```python
from build123d import *

# Parameters (mm, degrees)
F0_W     = 40
F0_H     = 20
F0_R     = 7.096656
F1_DEPTH = 25
F2_R     = 5
F3_DEPTH = 25


with BuildPart() as f1:
    # F0 (on Top) → F1 (new body)
    with BuildSketch(Plane.XY):
        with BuildLine():
            ThreePointArc((-133.453285, 45.853535), (-140.524353, 42.924603), (-143.453285, 35.853535))
            Line((-143.453285, 35.853535), (-143.453285, -36.596949))
            ThreePointArc((-143.453285, -36.596949), (-140.524353, -43.668016), (-133.453285, -46.596949))
            Line((-133.453285, -46.596949), (-93.023613, -46.596949))
            Line((-93.023613, -46.596949), (-93.023613, -53.490194))
            ThreePointArc((-93.023613, -53.490194), (-90.680467, -59.147049), (-85.023613, -61.490194))
            Line((-85.023613, -61.490194), (12.305611, -61.490194))
            Line((12.305611, -61.490194), (12.305611, -52.104292))
            Line((12.305611, -52.104292), (35.921164, -52.104292))
            ThreePointArc((35.921164, -52.104292), (39.456698, -50.639826), (40.921164, -47.104292))
            Line((40.921164, -47.104292), (40.921164, 45.453855))
            ThreePointArc((40.921164, 45.453855), (39.456698, 48.989389), (35.921164, 50.453855))
            Line((35.921164, 50.453855), (12.305611, 50.453855))
            Line((12.305611, 50.453855), (12.305611, 69.478564))
            Line((12.305611, 69.478564), (-88.023613, 69.478564))
            ThreePointArc((-88.023613, 69.478564), (-91.559147, 68.014098), (-93.023613, 64.478564))
            Line((-93.023613, 64.478564), (-93.023613, 45.853535))
            Line((-93.023613, 45.853535), (-133.453285, 45.853535))
        make_face()
        with BuildLine():
            Line((-138.153107, -41.573759), (-138.153107, -21.573759))
            Line((-138.153107, -21.573759), (-98.153107, -21.573759))
            Line((-98.153107, -21.573759), (-98.153107, -38.573759))
            ThreePointArc((-98.153107, -38.573759), (-99.031787, -40.695079), (-101.153107, -41.573759))
            Line((-101.153107, -41.573759), (-138.153107, -41.573759))
        make_face(mode=Mode.SUBTRACT)
        with Locations((-118.975651, -3.308505)):
            Rectangle(F0_W, F0_H, mode=Mode.SUBTRACT)
        with Locations((26.162848, -33.166352)):
            Circle(F0_R, mode=Mode.SUBTRACT)
        with BuildLine():
            Line((-76.998904, -36.091934), (-76.998904, 0))
            Line((-76.998904, 0), (0, 0))
            Line((0, 0), (0, -36.091934))
            ThreePointArc((0, -36.091934), (-1.464466, -39.627468), (-5, -41.091934))
            Line((-5, -41.091934), (-71.998904, -41.091934))
            ThreePointArc((-71.998904, -41.091934), (-75.534438, -39.627468), (-76.998904, -36.091934))
        make_face(mode=Mode.SUBTRACT)
        with Locations((25.7, 0.3)):
            Circle(F0_R, mode=Mode.SUBTRACT)
        with BuildLine():
            Line((-138.975651, 11.789608), (-138.975651, 31.789608))
            Line((-138.975651, 31.789608), (-103.975651, 31.789608))
            ThreePointArc((-103.975651, 31.789608), (-100.440117, 30.325142), (-98.975651, 26.789608))
            Line((-98.975651, 26.789608), (-98.975651, 11.789608))
            Line((-98.975651, 11.789608), (-138.975651, 11.789608))
        make_face(mode=Mode.SUBTRACT)
        with BuildLine():
            ThreePointArc((-77.227831, 41.128273), (-75.763365, 44.663807), (-72.227831, 46.128273))
            Line((-72.227831, 46.128273), (-5, 46.128273))
            ThreePointArc((-5, 46.128273), (-1.464466, 44.663807), (0, 41.128273))
            Line((0, 41.128273), (0, 17.970568))
            Line((0, 17.970568), (-77.227831, 17.970568))
            Line((-77.227831, 17.970568), (-77.227831, 41.128273))
        make_face(mode=Mode.SUBTRACT)
        with Locations((25.237152, 33.766352)):
            Circle(F0_R, mode=Mode.SUBTRACT)
    extrude(amount=F1_DEPTH)

    # F2
    f2_edges = [f1.edges().sort_by_distance(p)[0] for p in [
        (12.305611, -61.490194, 12.5),
        (-85.023613, -61.490194, 12.5),
    ]]
    fillet(f2_edges, radius=F2_R)

    # F0 (on Top) → F3 (join)
    with BuildSketch(Plane.XY):
        with BuildLine():
            ThreePointArc((-133.453285, 45.853535), (-140.524353, 42.924603), (-143.453285, 35.853535))
            Line((-143.453285, 35.853535), (-143.453285, -36.596949))
            ThreePointArc((-143.453285, -36.596949), (-140.524353, -43.668016), (-133.453285, -46.596949))
            Line((-133.453285, -46.596949), (-93.023613, -46.596949))
            Line((-93.023613, -46.596949), (-93.023613, -53.490194))
            ThreePointArc((-93.023613, -53.490194), (-90.680467, -59.147049), (-85.023613, -61.490194))
            Line((-85.023613, -61.490194), (12.305611, -61.490194))
            Line((12.305611, -61.490194), (12.305611, -52.104292))
            Line((12.305611, -52.104292), (35.921164, -52.104292))
            ThreePointArc((35.921164, -52.104292), (39.456698, -50.639826), (40.921164, -47.104292))
            Line((40.921164, -47.104292), (40.921164, 45.453855))
            ThreePointArc((40.921164, 45.453855), (39.456698, 48.989389), (35.921164, 50.453855))
            Line((35.921164, 50.453855), (12.305611, 50.453855))
            Line((12.305611, 50.453855), (12.305611, 69.478564))
            Line((12.305611, 69.478564), (-88.023613, 69.478564))
            ThreePointArc((-88.023613, 69.478564), (-91.559147, 68.014098), (-93.023613, 64.478564))
            Line((-93.023613, 64.478564), (-93.023613, 45.853535))
            Line((-93.023613, 45.853535), (-133.453285, 45.853535))
        make_face()
        with BuildLine():
            Line((-138.153107, -41.573759), (-138.153107, -21.573759))
            Line((-138.153107, -21.573759), (-98.153107, -21.573759))
            Line((-98.153107, -21.573759), (-98.153107, -38.573759))
            ThreePointArc((-98.153107, -38.573759), (-99.031787, -40.695079), (-101.153107, -41.573759))
            Line((-101.153107, -41.573759), (-138.153107, -41.573759))
        make_face(mode=Mode.SUBTRACT)
        with Locations((-118.975651, -3.308505)):
            Rectangle(F0_W, F0_H, mode=Mode.SUBTRACT)
        with Locations((26.162848, -33.166352)):
            Circle(F0_R, mode=Mode.SUBTRACT)
        with BuildLine():
            Line((-76.998904, -36.091934), (-76.998904, 0))
            Line((-76.998904, 0), (0, 0))
            Line((0, 0), (0, -36.091934))
            ThreePointArc((0, -36.091934), (-1.464466, -39.627468), (-5, -41.091934))
            Line((-5, -41.091934), (-71.998904, -41.091934))
            ThreePointArc((-71.998904, -41.091934), (-75.534438, -39.627468), (-76.998904, -36.091934))
        make_face(mode=Mode.SUBTRACT)
        with Locations((25.7, 0.3)):
            Circle(F0_R, mode=Mode.SUBTRACT)
        with BuildLine():
            Line((-138.975651, 11.789608), (-138.975651, 31.789608))
            Line((-138.975651, 31.789608), (-103.975651, 31.789608))
            ThreePointArc((-103.975651, 31.789608), (-100.440117, 30.325142), (-98.975651, 26.789608))
            Line((-98.975651, 26.789608), (-98.975651, 11.789608))
            Line((-98.975651, 11.789608), (-138.975651, 11.789608))
        make_face(mode=Mode.SUBTRACT)
        with BuildLine():
            ThreePointArc((-77.227831, 41.128273), (-75.763365, 44.663807), (-72.227831, 46.128273))
            Line((-72.227831, 46.128273), (-5, 46.128273))
            ThreePointArc((-5, 46.128273), (-1.464466, 44.663807), (0, 41.128273))
            Line((0, 41.128273), (0, 17.970568))
            Line((0, 17.970568), (-77.227831, 17.970568))
            Line((-77.227831, 17.970568), (-77.227831, 41.128273))
        make_face(mode=Mode.SUBTRACT)
        with Locations((25.237152, 33.766352)):
            Circle(F0_R, mode=Mode.SUBTRACT)
    extrude(amount=F3_DEPTH)


solid = f1.part
```
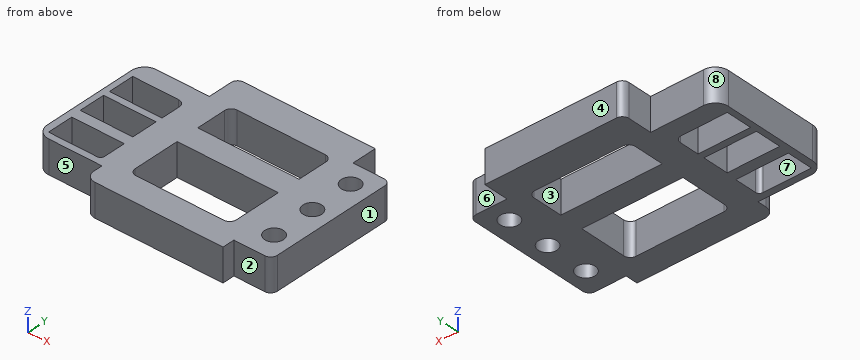
The listing builds one solid part. Answer for the finished solid, in the listing's coordinates (mm). Face numbers are marked on the shaded views. A direction names the side the tool comes from. Coordinates: 2 decimals unless noted, no trailing zeros. Write each loop counter-clockwise with the first axis right and the second up, starting at its lowest first coordinate (ties: lowest second). Pieces come first, ordered by that corner, then holes. Notation, with made-up numbers: (20.25, 69.5) - (66.25, 69.5) arc R13 cw to (66.25, 74.5) - close; hole circle Ø2 at (35.5, 80). An arc over 180 degrees is marked (long way). Return JSON: item names as keys, results as strings. Group by question number.
1. A cutting plane is placed at C-C, the plane y = 56.5. Determine the outline of the cut face in (x, z), plus the area to 3 significant figures.
2. A cutting plane is placed at D-D, the plane x = 25.7. Determine the outline of the cut face in (y, z), plus the area to 3 significant figures.
3. Straight lines are drawn through the part: L1, parallel to Y at x = 25.7, z = 11.5; L2, parallel to Y at x = -38, z = 1.25; L3, parallel to X at y = 2.5, z = 15.25. For each, find the intervals that lie inside material, in ascending order.
4. A cutting plane is placed at B-B, the plane y = 39. Determine the outline of the cut face in (x, z).
5. Which of the six approach directions +Z, -Z, +X, -X, +Y, -Y give full straight-line access (tool end or side, diameter ignored) to the marked faces 4, 5, 6, 7 and 8?
6. Determine the mould class of the marked faces 1, 2 and 3 for opening direction X: released by +X, released by -X, zero draft, split by the parting line, or undercut.
7. Given pin 1 (12.5 mm diameter, centred on x = -128, z = 17.5, fed in from -Y); pin 2 (7.5 mm diameter, centred on x = -126, z = 7.5, fed in from +Y); pin 3 (3 mm diameter, centred on y = -46.5, z = 11.5, fed in from -X); pin 4 (8.5 mm diameter, centred on x = 25.7, y = 0.3, fed in from +Z), each flat-ended and moving along its own axis, determine where each tip first touches the part or whether it passes through.
8. A cutting plane is placed at A-A, the plane x = -121. Determine the outline of the cut face in (y, z), plus the area to 3 significant figures.
Ans:
{
 "1": {"outline": "(-93.02, 0) - (12.31, 0) - (12.31, 25) - (-93.02, 25) - close", "area": "2,630 mm²"},
 "2": {"outline": "(-52.1, 0) - (-40.25, 0) - (-40.25, 25) - (-52.1, 25) - close; (-26.08, 0) - (-6.8, 0) - (-6.8, 25) - (-26.08, 25) - close; (7.4, 0) - (26.68, 0) - (26.68, 25) - (7.4, 25) - close; (40.85, 0) - (50.45, 0) - (50.45, 25) - (40.85, 25) - close", "area": "1,500 mm²"},
 "3": {"L1": "-52.1 to -40.25, -26.08 to -6.8, 7.4 to 26.68, 40.85 to 50.45", "L2": "-61.49 to -41.09, 0 to 17.97, 46.13 to 69.48", "L3": "-143.45 to -138.98, -98.98 to 18.95, 32.45 to 40.92"},
 "4": {"outline": "(-142.95, 0) - (-77.23, 0) - (-77.23, 25) - (-142.95, 25) - close; (0, 0) - (20.44, 0) - (20.44, 25) - (0, 25) - close; (30.03, 0) - (40.92, 0) - (40.92, 25) - (30.03, 25) - close"},
 "5": {"face 4": "+Z, -Z, +X, -X, +Y", "face 5": "+Z, -Z, -X, -Y", "face 6": "+Z, -Z, +X, +Y", "face 7": "+Z, -Z", "face 8": "+Z, -Z, -X, +Y"},
 "6": {"face 1": "released by +X", "face 2": "zero draft", "face 3": "undercut"},
 "7": {"pin 1": "y = -46.6", "pin 2": "y = 45.85", "pin 3": "x = -138.87", "pin 4": "through"},
 "8": {"outline": "(-46.6, 0) - (-41.57, 0) - (-41.57, 25) - (-46.6, 25) - close; (-21.57, 0) - (-13.31, 0) - (-13.31, 25) - (-21.57, 25) - close; (6.69, 0) - (11.79, 0) - (11.79, 25) - (6.69, 25) - close; (31.79, 0) - (45.85, 0) - (45.85, 25) - (31.79, 25) - close", "area": "811 mm²"}
}
